Input: part model. Units: mm. Frame: model coordinates. Face numbers are marked on the shaded views. Give positions to 0.01 mm unless a question says otherwise; leave off trailing zeros. Order: outer loops, then holes, each group sorted by start corner. A loop starts at its lowest first (then second) coordinate and runs counter-clockwise, first axis right, second up. Notation, with made-up numbers: (63.5, 7.5) -> (101.5, 7.5) arc R18 cw to (101.5, 24.5) -> close; hole circle Ø1 at (14.5, -32.5). An arc over 180 degrees is marked (long way). Use a Markdown table: item, result. Add a question column.
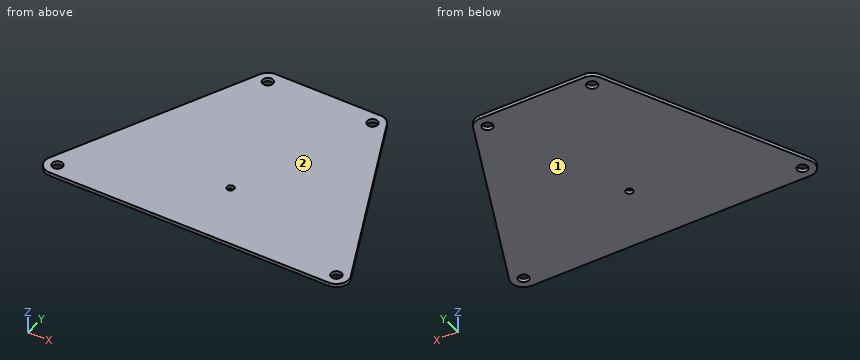
Autodesk Inventor part; units mm, degrees
ref_plane "YZ Plane" through (0, 0, 0) normal (1, 0, 0) x (0, 1, 0)
ref_plane "XZ Plane" through (0, 0, 0) normal (0, 1, 0) x (-1, 0, 0)
ref_plane "XY Plane" through (0, 0, 0) normal (0, 0, 1) x (1, 0, 0)
sketch "Sketch1" plane through (0, 0, 0) normal (0, 0, 1) x (1, 0, 0)
  circle A0 centre (50, 110) radius 3
  circle A1 centre (0, 0) radius 3
  circle A2 centre (160, 0) radius 3
  circle A3 centre (80, 30) radius 2.05
  arc A4 (50, 117) -> (43.6274, 112.8966) centre (50, 110) ccw
  circle A5 centre (110, 110) radius 3
  arc A6 (116.3726, 112.8966) -> (110, 117) centre (110, 110) ccw
  arc A7 (-6.3726, 2.8966) -> (0, -7) centre (0, 0) ccw
  arc A8 (160, -7) -> (166.3726, 2.8966) centre (160, 0) ccw
  line L0 (-6.3726, 2.8966) -> (43.6274, 112.8966)
  line L1 (50, 117) -> (110, 117)
  line L2 (166.3726, 2.8966) -> (116.3726, 112.8966)
  line L3 (0, -7) -> (160, -7)
  dimension "d7" = 6
  dimension "d9" = 6
  dimension "d10" = 6
  dimension "d11" = 4.1
  dimension "d12" = 14
  dimension "d13" = 6
  dimension "d14" = 14
  dimension "d15" = 14
  dimension "d16" = 14
  dimension "d25" = 160
  dimension "d26" = 60
  dimension "d27" = 110
  dimension "d28" = 30
extrude "Extrusion1" add sketch "Sketch1" along normal blind 2
properties part number "Frame" material "Steel, Mild"
Q1. Section query B-B (y = 0). Return loops of the section in (x, z).
Q2. Section query A-A (x = 80). Return loops of the section in (y, z), plus the area to 3 significant figures.
Q3. Draft query along Z for the marked faces 1 and 2. Return one class per face: +Z half, -Z half, draft (parallel to the pull), parting line (faces both ways), or undercut.
Q4. Section query C-C (z = 0.5). Return loops of the section in (x, y).
Q5. First-contact query: pin 1 (1 mm diameter, centred on x = 135, z = 1, fed in from +Y); pin 2 (1 mm diameter, centred on y = 76.5, z = 1, fed in from -X). Flat tips, straight axial feed; report the tip coordinate or a pass-through.
Q6. Section query D-D (y = 30). Return loops of the section in (x, z), plus the area to 3 significant figures.
Q7. Ray query, line 1 (Y direction, x = 80, z = 1.3); line 2 (Y direction, x = 110, z = 1.2); line 3 (X direction, y = 93.5, z = 0.35). Return the intervals inside material, ascending.
Solution:
| question | item | result |
|---|---|---|
| 1 | outline | (-7, 0) -> (-3, 0) -> (-3, 2) -> (-7, 2) -> close; (3, 0) -> (157, 0) -> (157, 2) -> (3, 2) -> close; (163, 0) -> (167, 0) -> (167, 2) -> (163, 2) -> close |
| 2 | outline | (-7, 0) -> (27.95, 0) -> (27.95, 2) -> (-7, 2) -> close; (32.05, 0) -> (117, 0) -> (117, 2) -> (32.05, 2) -> close |
| 2 | area | 240 mm² |
| 3 | face 1 | -Z half |
| 3 | face 2 | +Z half |
| 4 | outline | (-6.37, 2.9) arc R7 ccw to (0, -7) -> (160, -7) arc R7 ccw to (166.37, 2.9) -> (116.37, 112.9) arc R7 ccw to (110, 117) -> (50, 117) arc R7 ccw to (43.63, 112.9) -> close; hole circle Ø6 at (0, 0); hole circle Ø6 at (50, 110); hole circle Ø4.1 at (80, 30); hole circle Ø6 at (110, 110); hole circle Ø6 at (160, 0) |
| 5 | pin 1 | stops at y = 73.02 |
| 5 | pin 2 | stops at x = 26.86 |
| 6 | outline | (5.95, 0) -> (77.95, 0) -> (77.95, 2) -> (5.95, 2) -> close; (82.05, 0) -> (154.05, 0) -> (154.05, 2) -> (82.05, 2) -> close |
| 6 | area | 288 mm² |
| 7 | line 1 | y = -7 to 27.95, 32.05 to 117 |
| 7 | line 2 | y = -7 to 107, 113 to 117 |
| 7 | line 3 | x = 34.81 to 125.19 |
